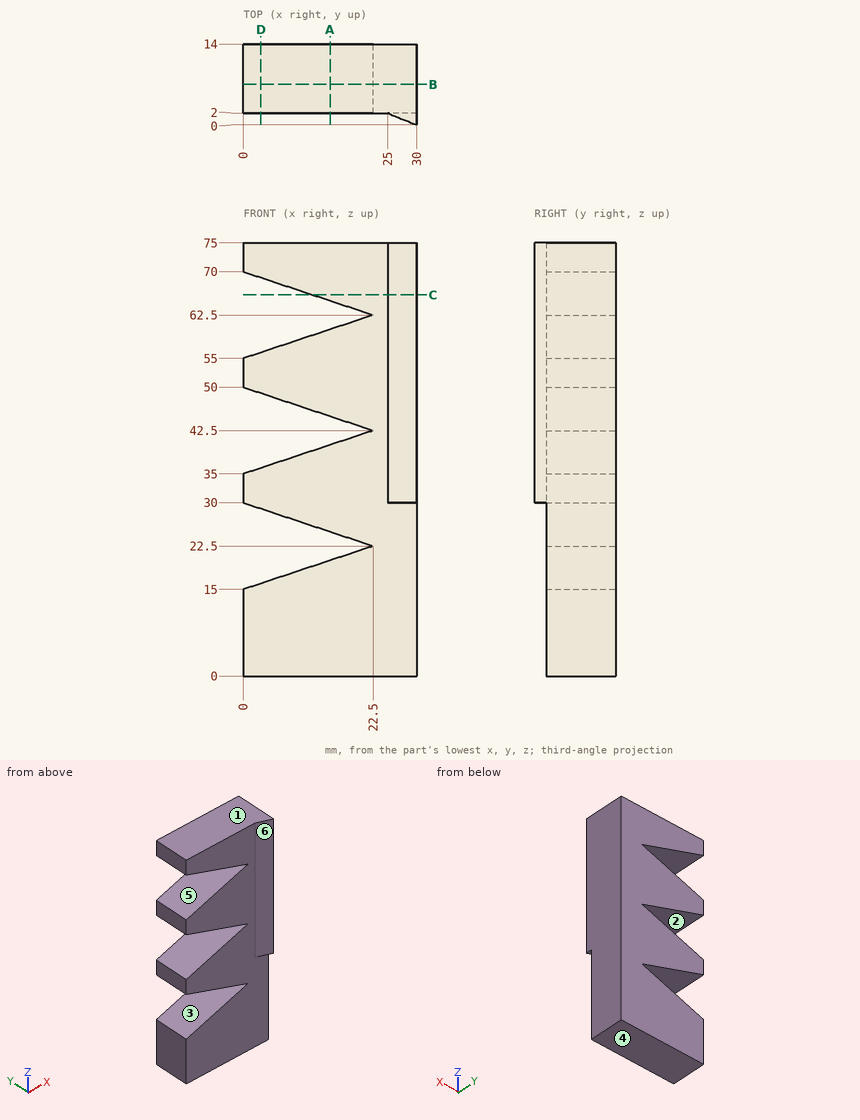
Could you check a few things on this drawing? It's one solid part, dimensions in mm from its lowest x, y, z. A direction names the side the tool comes from. Coordinates: 2 decimals unless noted, no trailing zeros. Order: outer loops, then holes, each group sorted by start corner. A loop starts at its lowest first (then second) coordinate and runs counter-clockwise, first axis right, second up. Notation, with made-up numbers: (20, 1) - (35, 1) arc R19 ccw to (35, 17) - close; hole circle Ø9 at (72.5, 63). An arc over 180 degrees is marked (long way). One line per question, with ' | ' between items. Start each with the question number.
1. If we section it at D-D (x = 3): Write out the boundary of the cut face in (y, z).
2. Which directions (+Z, -Z, +X, -X, +Y, -Y) give clear straight access to the entire face, cutting with the end or side of a thin tool? Please do the marked faces 5 and 6.
3. I'm going to push flat-ended pins straight in: pin 1 Ø1 at (x, z) = (4, 14.5) entering from -Y; pin 2 Ø1 at (x, z) = (13, 64.5) entering from -Y; pin 3 Ø5 at (x, y) = (14.5, 6.5) entering from -Z. Where does each tip first touch, or does it pass through?
4. Please list where these lines run through material, in increasing order: line 1 along Z through (x, y) = (19, 13.75); line 2 along Z through (x, y) = (5.25, 4.5); line 3 along Y through (x, z) = (20.5, 49). Write a range as [from, to].
5. If we section it at A-A (x = 15): Write out the boundary of the cut face in (y, z), and give its area (3 significant figures).
6. If we mould it in two halves opening along Z, with no side actions, what happens to the marked faces 1, 2, 3 and 4? For each: released by +Z, released by -Z, zero draft, split by the parting line, or undercut.
7. If we section it at C-C (z = 66): Write out the boundary of the cut face in (x, y), and give its area (3 significant figures).
8. If we section it at B-B (y = 7): Write out the boundary of the cut face in (x, z).
Model answer:
1) outline: (2, 0) - (14, 0) - (14, 16) - (2, 16) - close; (2, 29) - (14, 29) - (14, 36) - (2, 36) - close; (2, 49) - (14, 49) - (14, 56) - (2, 56) - close; (2, 69) - (14, 69) - (14, 75) - (2, 75) - close
2) face 5: -X, +Y, -Y | face 6: +Z, -Z, -X, -Y
3) pin 1: stops at y = 2 | pin 2: passes through | pin 3: stops at z = 0
4) line 1: z = [0, 21.33], [23.67, 41.33], [43.67, 61.33], [63.67, 75] | line 2: z = [0, 16.75], [28.25, 36.75], [48.25, 56.75], [68.25, 75] | line 3: y = [2, 14]
5) outline: (2, 0) - (14, 0) - (14, 20) - (2, 20) - close; (2, 25) - (14, 25) - (14, 40) - (2, 40) - close; (2, 45) - (14, 45) - (14, 60) - (2, 60) - close; (2, 65) - (14, 65) - (14, 75) - (2, 75) - close | area: 720 mm²
6) face 1: released by +Z | face 2: undercut | face 3: undercut | face 4: released by -Z
7) outline: (12, 2) - (25, 2) - (30, 0) - (30, 14) - (12, 14) - close | area: 221 mm²
8) outline: (0, 0) - (30, 0) - (30, 75) - (0, 75) - (0, 70) - (22.5, 62.5) - (0, 55) - (0, 50) - (22.5, 42.5) - (0, 35) - (0, 30) - (22.5, 22.5) - (0, 15) - close
